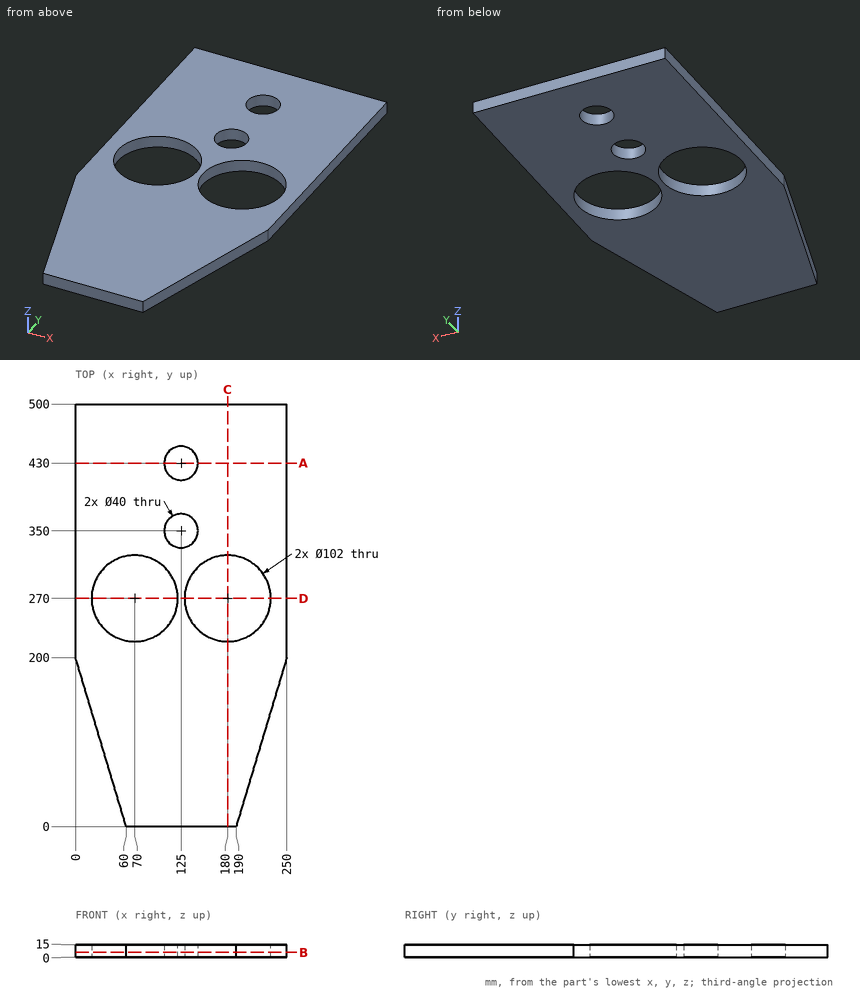
Geometry check sheet. Reference: drawing and pictorial views, mm from the part's lowest x, y, z. Coordinates: 2 decimals unless noted, no trailing zeros. Order: outer loops, then holes, each group sorted by start corner. A loop starts at its lowest first (then second) coordinate and runs counter-clockwise, first axis right, second up.
Item 1: Depth check by flat-ended pin: pin 1 (8 mm diameter, centred on x = 65.5, z = 4, fed in from -Y); pin 2 (6 mm diameter, centred on y = 105, z = 2.5, fed in from +X); pin 3 (6 mm diameter, centred on y = 69.5, z = 12, fed in from -X). Enter the tip coordinate at first touch or a pass-through.
Item 2: Scan lines: line 1 along Y through (x, z) = (125, 10.75); line 2 along Y through (x, z) = (113, 8.5); line 3 along Y through (x, z) = (70, 11.25). Record each from-to range of solid material in increasing order.
Item 3: Section check B-B (z = 6). Enter the section's corners in (x, y), plus the area to 3 significant figures.
Item 4: Section check A-A (y = 430). Enter the section's corners in (x, z).
Item 5: Section check D-D (y = 270). Enter the section's corners in (x, z).
Item 6: Section check C-C (x = 180). Enter the section's corners in (y, z), plus the area to 3 significant figures.
Check sheet entries:
1. pin 1: stops at y = 0
1. pin 2: stops at x = 222.4
1. pin 3: stops at x = 38.25
2. line 1: y = 0 to 330, 370 to 410, 450 to 500
2. line 2: y = 0 to 242.58, 297.42 to 334, 366 to 414, 446 to 500
2. line 3: y = 0 to 219, 321 to 500
3. outline: (0, 200) - (60, 0) - (190, 0) - (250, 200) - (250, 500) - (0, 500) - close; hole circle Ø102 at (70, 270); hole circle Ø40 at (125, 350); hole circle Ø40 at (125, 430); hole circle Ø102 at (180, 270)
3. area: 94,100 mm2
4. outline: (0, 0) - (105, 0) - (105, 15) - (0, 15) - close; (145, 0) - (250, 0) - (250, 15) - (145, 15) - close
5. outline: (0, 0) - (19, 0) - (19, 15) - (0, 15) - close; (121, 0) - (129, 0) - (129, 15) - (121, 15) - close; (231, 0) - (250, 0) - (250, 15) - (231, 15) - close
6. outline: (0, 0) - (219, 0) - (219, 15) - (0, 15) - close; (321, 0) - (500, 0) - (500, 15) - (321, 15) - close
6. area: 5,970 mm2
